Read the model definition and answer for the solid it produces. Units are mm, in the model's axes. A direction names the side the tool comes from. Give positions to 0.01 mm unless a question says otherwise; leave off trailing zeros. Loops run counter-clockwise (first coordinate to the right, second up) from the corner with the lowest first, then second, coordinate; pieces in that order, holes last. Notation, with made-up numbers: (20, 30.25) - (36, 30.25) arc R31 ccw to (36, 69.25) - close; hole circle Ø2 at (52.5, 73.5). An arc over 180 degrees is marked (long way). Write item = value, one per line. Start each with the question number.
from build123d import *

# Parameters (mm, degrees)
F1_DEPTH      = 20
F2_DEPTH      = 1.93
F3_DEPTH      = 3
F4_R          = 1.5
F5_DEPTH      = 7
F5_DEPTH_BACK = 7


with BuildPart() as f1:
    # F0 (on Front) → F1 (new body)
    with BuildSketch(Plane.XZ):
        with BuildLine():
            Line((0, 0), (3.9, 0))
            ThreePointArc((3.9, 0), (3.7194961079, 1.1727526181), (3.1946929727, 2.2369481018))
            Line((3.1946929727, 2.2369481018), (0, 0))
        make_face()
        with BuildLine():
            Line((0, 0), (3.1946929727, 2.2369481018))
            ThreePointArc((3.1946929727, 2.2369481018), (2.9875733282, 2.5068716778), (2.7577164466, 2.7577164466))
            Line((2.7577164466, 2.7577164466), (0, 0))
        make_face()
        with BuildLine():
            Line((2.2369481018, 3.1946929727), (0, 0))
            Line((0, 0), (2.7577164466, 2.7577164466))
            ThreePointArc((2.7577164466, 2.7577164466), (2.5068716778, 2.9875733282), (2.2369481018, 3.1946929727))
        make_face()
        with BuildLine():
            Line((0.6772278929, 3.8407502367), (0, 0))
            Line((0, 0), (2.2369481018, 3.1946929727))
            ThreePointArc((2.2369481018, 3.1946929727), (1.4924653862, 3.6031301768), (0.6772278929, 3.8407502367))
        make_face()
        with BuildLine():
            Line((0, 3.9), (0, 0))
            Line((0, 0), (0.6772278929, 3.8407502367))
            ThreePointArc((0.6772278929, 3.8407502367), (0.3399073967, 3.8851593226), (0, 3.9))
        make_face()
        with BuildLine():
            Line((-0.6772278929, 3.8407502367), (0, 0))
            Line((0, 0), (0, 3.9))
            ThreePointArc((0, 3.9), (-0.3399073967, 3.8851593226), (-0.6772278929, 3.8407502367))
        make_face()
        with BuildLine():
            Line((-2.2369481018, 3.1946929727), (0, 0))
            Line((0, 0), (-0.6772278929, 3.8407502367))
            ThreePointArc((-0.6772278929, 3.8407502367), (-1.4924653862, 3.6031301768), (-2.2369481018, 3.1946929727))
        make_face()
        with BuildLine():
            Line((-2.7577164466, 2.7577164466), (0, 0))
            Line((0, 0), (-2.2369481018, 3.1946929727))
            ThreePointArc((-2.2369481018, 3.1946929727), (-2.5068716778, 2.9875733282), (-2.7577164466, 2.7577164466))
        make_face()
        with BuildLine():
            Line((-3.1946929727, 2.2369481018), (0, 0))
            Line((0, 0), (-2.7577164466, 2.7577164466))
            ThreePointArc((-2.7577164466, 2.7577164466), (-2.9875733282, 2.5068716778), (-3.1946929727, 2.2369481018))
        make_face()
        with BuildLine():
            ThreePointArc((-3.1946929727, 2.2369481018), (-3.7194961079, 1.1727526181), (-3.9, 0))
            Line((-3.9, 0), (0, 0))
            Line((0, 0), (-3.1946929727, 2.2369481018))
        make_face()
        with BuildLine():
            ThreePointArc((-3.9, 0), (0, -3.9), (3.9, 0))
            Line((3.9, 0), (0, 0))
            Line((0, 0), (-3.9, 0))
        make_face()
        with BuildLine():
            ThreePointArc((3.1946929727, 2.2369481018), (3.7194961079, 1.1727526181), (3.9, 0))
            Line((3.9, 0), (5, 0))
            ThreePointArc((5, 0), (4.7685847537, 1.5035289975), (4.0957602214, 2.8678821818))
            Line((4.0957602214, 2.8678821818), (3.1946929727, 2.2369481018))
        make_face()
        with BuildLine():
            ThreePointArc((2.7577164466, 2.7577164466), (2.9875733282, 2.5068716778), (3.1946929727, 2.2369481018))
            Line((3.1946929727, 2.2369481018), (4.0957602214, 2.8678821818))
            ThreePointArc((4.0957602214, 2.8678821818), (3.8302222156, 3.2139380484), (3.5355339059, 3.5355339059))
            Line((3.5355339059, 3.5355339059), (2.7577164466, 2.7577164466))
        make_face()
        with BuildLine():
            ThreePointArc((2.2369481018, 3.1946929727), (2.5068716778, 2.9875733282), (2.7577164466, 2.7577164466))
            Line((2.7577164466, 2.7577164466), (3.5355339059, 3.5355339059))
            ThreePointArc((3.5355339059, 3.5355339059), (3.2139380484, 3.8302222156), (2.8678821818, 4.0957602214))
            Line((2.8678821818, 4.0957602214), (2.2369481018, 3.1946929727))
        make_face()
        with BuildLine():
            ThreePointArc((0.6772278929, 3.8407502367), (1.4924653862, 3.6031301768), (2.2369481018, 3.1946929727))
            Line((2.2369481018, 3.1946929727), (2.8678821818, 4.0957602214))
            ThreePointArc((2.8678821818, 4.0957602214), (1.9134171618, 4.6193976626), (0.8682408883, 4.9240387651))
            Line((0.8682408883, 4.9240387651), (0.6772278929, 3.8407502367))
        make_face()
        with BuildLine():
            Line((0, 5), (0, 3.9))
            ThreePointArc((0, 3.9), (0.3399073967, 3.8851593226), (0.6772278929, 3.8407502367))
            Line((0.6772278929, 3.8407502367), (0.8682408883, 4.9240387651))
            ThreePointArc((0.8682408883, 4.9240387651), (0.4357787137, 4.9809734905), (0, 5))
        make_face()
        with BuildLine():
            ThreePointArc((-0.6772278929, 3.8407502367), (-0.3399073967, 3.8851593226), (0, 3.9))
            Line((0, 3.9), (0, 5))
            ThreePointArc((0, 5), (-0.4357787137, 4.9809734905), (-0.8682408883, 4.9240387651))
            Line((-0.8682408883, 4.9240387651), (-0.6772278929, 3.8407502367))
        make_face()
        with BuildLine():
            ThreePointArc((-2.2369481018, 3.1946929727), (-1.4924653862, 3.6031301768), (-0.6772278929, 3.8407502367))
            Line((-0.6772278929, 3.8407502367), (-0.8682408883, 4.9240387651))
            ThreePointArc((-0.8682408883, 4.9240387651), (-1.9134171618, 4.6193976626), (-2.8678821818, 4.0957602214))
            Line((-2.8678821818, 4.0957602214), (-2.2369481018, 3.1946929727))
        make_face()
        with BuildLine():
            Line((-3.5355339059, 3.5355339059), (-2.7577164466, 2.7577164466))
            ThreePointArc((-2.7577164466, 2.7577164466), (-2.5068716778, 2.9875733282), (-2.2369481018, 3.1946929727))
            Line((-2.2369481018, 3.1946929727), (-2.8678821818, 4.0957602214))
            ThreePointArc((-2.8678821818, 4.0957602214), (-3.2139380484, 3.8302222156), (-3.5355339059, 3.5355339059))
        make_face()
        with BuildLine():
            Line((-4.0957602214, 2.8678821818), (-3.1946929727, 2.2369481018))
            ThreePointArc((-3.1946929727, 2.2369481018), (-2.9875733282, 2.5068716778), (-2.7577164466, 2.7577164466))
            Line((-2.7577164466, 2.7577164466), (-3.5355339059, 3.5355339059))
            ThreePointArc((-3.5355339059, 3.5355339059), (-3.8302222156, 3.2139380484), (-4.0957602214, 2.8678821818))
        make_face()
        with BuildLine():
            Line((-5, 0), (-3.9, 0))
            ThreePointArc((-3.9, 0), (-3.7194961079, 1.1727526181), (-3.1946929727, 2.2369481018))
            Line((-3.1946929727, 2.2369481018), (-4.0957602214, 2.8678821818))
            ThreePointArc((-4.0957602214, 2.8678821818), (-4.7685847537, 1.5035289975), (-5, 0))
        make_face()
        with BuildLine():
            Line((5, 0), (3.9, 0))
            ThreePointArc((3.9, 0), (0, -3.9), (-3.9, 0))
            Line((-3.9, 0), (-5, 0))
            ThreePointArc((-5, 0), (0, -5), (5, 0))
        make_face()
    extrude(amount=F1_DEPTH)

    # F0 (on Front) → F2 (cut)
    with BuildSketch(Plane.XZ):
        with BuildLine():
            Line((0, 0), (3.9, 0))
            ThreePointArc((3.9, 0), (3.7194961079, 1.1727526181), (3.1946929727, 2.2369481018))
            Line((3.1946929727, 2.2369481018), (0, 0))
        make_face()
        with BuildLine():
            Line((0, 0), (3.1946929727, 2.2369481018))
            ThreePointArc((3.1946929727, 2.2369481018), (2.9875733282, 2.5068716778), (2.7577164466, 2.7577164466))
            Line((2.7577164466, 2.7577164466), (0, 0))
        make_face()
        with BuildLine():
            Line((2.2369481018, 3.1946929727), (0, 0))
            Line((0, 0), (2.7577164466, 2.7577164466))
            ThreePointArc((2.7577164466, 2.7577164466), (2.5068716778, 2.9875733282), (2.2369481018, 3.1946929727))
        make_face()
        with BuildLine():
            Line((0.6772278929, 3.8407502367), (0, 0))
            Line((0, 0), (2.2369481018, 3.1946929727))
            ThreePointArc((2.2369481018, 3.1946929727), (1.4924653862, 3.6031301768), (0.6772278929, 3.8407502367))
        make_face()
        with BuildLine():
            Line((0, 3.9), (0, 0))
            Line((0, 0), (0.6772278929, 3.8407502367))
            ThreePointArc((0.6772278929, 3.8407502367), (0.3399073967, 3.8851593226), (0, 3.9))
        make_face()
        with BuildLine():
            Line((-0.6772278929, 3.8407502367), (0, 0))
            Line((0, 0), (0, 3.9))
            ThreePointArc((0, 3.9), (-0.3399073967, 3.8851593226), (-0.6772278929, 3.8407502367))
        make_face()
        with BuildLine():
            Line((-2.2369481018, 3.1946929727), (0, 0))
            Line((0, 0), (-0.6772278929, 3.8407502367))
            ThreePointArc((-0.6772278929, 3.8407502367), (-1.4924653862, 3.6031301768), (-2.2369481018, 3.1946929727))
        make_face()
        with BuildLine():
            Line((-2.7577164466, 2.7577164466), (0, 0))
            Line((0, 0), (-2.2369481018, 3.1946929727))
            ThreePointArc((-2.2369481018, 3.1946929727), (-2.5068716778, 2.9875733282), (-2.7577164466, 2.7577164466))
        make_face()
        with BuildLine():
            Line((-3.1946929727, 2.2369481018), (0, 0))
            Line((0, 0), (-2.7577164466, 2.7577164466))
            ThreePointArc((-2.7577164466, 2.7577164466), (-2.9875733282, 2.5068716778), (-3.1946929727, 2.2369481018))
        make_face()
        with BuildLine():
            ThreePointArc((-3.1946929727, 2.2369481018), (-3.7194961079, 1.1727526181), (-3.9, 0))
            Line((-3.9, 0), (0, 0))
            Line((0, 0), (-3.1946929727, 2.2369481018))
        make_face()
        with BuildLine():
            ThreePointArc((-3.9, 0), (0, -3.9), (3.9, 0))
            Line((3.9, 0), (0, 0))
            Line((0, 0), (-3.9, 0))
        make_face()
    extrude(amount=F2_DEPTH, mode=Mode.SUBTRACT)

    # F0 (on Front) → F3 (join)
    with BuildSketch(Plane.XZ):
        with BuildLine():
            ThreePointArc((3.5355339059, 3.5355339059), (3.8302222156, 3.2139380484), (4.0957602214, 2.8678821818))
            Line((4.0957602214, 2.8678821818), (5.3244882879, 3.7282468363))
            ThreePointArc((5.3244882879, 3.7282468363), (4.5961940777, 4.5961940777), (3.7282468363, 5.3244882879))
            Line((3.7282468363, 5.3244882879), (2.8678821818, 4.0957602214))
            ThreePointArc((2.8678821818, 4.0957602214), (3.2139380484, 3.8302222156), (3.5355339059, 3.5355339059))
        make_face()
        with BuildLine():
            ThreePointArc((-0.8682408883, 4.9240387651), (-0.4357787137, 4.9809734905), (0, 5))
            ThreePointArc((0, 5), (0.4357787137, 4.9809734905), (0.8682408883, 4.9240387651))
            Line((0.8682408883, 4.9240387651), (1.1287131548, 6.4012503946))
            ThreePointArc((1.1287131548, 6.4012503946), (0, 6.5), (-1.1287131548, 6.4012503946))
            Line((-1.1287131548, 6.4012503946), (-0.8682408883, 4.9240387651))
        make_face()
        with BuildLine():
            Line((-5.3244882879, 3.7282468363), (-4.0957602214, 2.8678821818))
            ThreePointArc((-4.0957602214, 2.8678821818), (-3.8302222156, 3.2139380484), (-3.5355339059, 3.5355339059))
            ThreePointArc((-3.5355339059, 3.5355339059), (-3.2139380484, 3.8302222156), (-2.8678821818, 4.0957602214))
            Line((-2.8678821818, 4.0957602214), (-3.7282468363, 5.3244882879))
            ThreePointArc((-3.7282468363, 5.3244882879), (-4.5961940777, 4.5961940777), (-5.3244882879, 3.7282468363))
        make_face()
    extrude(amount=F3_DEPTH)

    # F4 (on Right) → F5 (join, two sides)
    with BuildSketch(Plane.YZ) as f5_sk:
        with Locations((-15, 0)):
            Circle(F4_R)
    extrude(amount=F5_DEPTH)
    extrude(f5_sk.sketch, amount=-F5_DEPTH_BACK)


solid = f1.part
1. A cutting plane is placed at D-D on y = -15. Give the vertices of the cut face in (x, z).
2. Consider line 1 along X through (y, z) = (-8.5, 1.5); line 2 along Y through (x, z) = (-0.5, 2.5). Determine where each line is inside the solid, lowest interval first. Write a range as [from, to].
3. Given P1, Ø1.7, axis at x = 0, z = 6, coming from the -Y side; P2, Ø1, axis at y = -10.5, z = 0, coming from the +X side; P3, Ø1, axis at x = -5.5, z = 3, coming from the -Y side; P4, Ø3, axis at y = -7.5, z = -3.5, coming from the +X side, each flat-ended and moving along its own axis, determine where each tip first touches the part or whether it passes through.
4. For a pull along X with two mould halves and no side action, classify faces 1 (the flat face through (0, -20, 0)), 2 (the cylindrical face through (0, -1.5, 6.5)), 3 (the flat face through (-1, -1.48, 5.67)), 4 (the flat face through (-7, -15, 0)) as released by +X, released by -X, zero draft, split by the parting line, or undercut.
5. A tool of negligible diameter and unlimited length cuts with its end or side. For faces 5 (the flat face through (4.7, -1.48, 3.29)), 6 (the cylindrical face through (5.869, -13.614, -0.575)), 7 (the flat face through (-4, -3, 4)), from which of +Z, -Z, +X, -X, +Y, -Y can it reach the whole face along a straight path? Write none if from no direction.
6. A cutting plane is placed at B-B on x = -1.5. Give the vertices of the cut face in (y, z).
7. A cutting plane is placed at C-C on y = -7. Give the vertices of the cut face in (x, z), and give its area (3 significant figures).
8. A cutting plane is placed at A-A on y = -1.25. Give the vertices of the cut face in (x, z).
Reply:
q1.outline = (-7, -1.5) - (-4.77, -1.5) arc R5 ccw to (4.77, -1.5) - (7, -1.5) - (7, 1.5) - (4.77, 1.5) arc R5 ccw to (-4.77, 1.5) - (-7, 1.5) - close
q2.line_1 = [-4.77, 4.77]
q2.line_2 = [-20, -1.93]
q3.P1 = -3
q3.P2 = 5
q3.P3 = through
q3.P4 = 4.58
q4.face_1 = zero draft
q4.face_2 = split by the parting line
q4.face_3 = undercut
q4.face_4 = released by -X
q5.face_5 = +X, +Y, -Y
q5.face_6 = +X
q5.face_7 = +Z, -X, -Y
q6.outline = (-20, -4.77) - (0, -4.77) - (0, -3.6) - (-1.93, -3.6) - (-1.93, 3.6) - (0, 3.6) - (0, 4.77) - (-20, 4.77) - close
q7.outline = circle Ø10 at (0, 0)
q7.area = 78.5 mm^2
q8.outline = (-5.32, 3.73) - (-4.1, 2.87) arc R5 ccw (long way) to (4.1, 2.87) - (5.32, 3.73) arc R6.5 ccw to (3.73, 5.32) - (2.87, 4.1) arc R5 ccw to (0.87, 4.92) - (1.13, 6.4) arc R6.5 ccw to (-1.13, 6.4) - (-0.87, 4.92) arc R5 ccw to (-2.87, 4.1) - (-3.73, 5.32) arc R6.5 ccw to start; hole circle Ø7.8 at (0, 0)
